Answer from the drawing. Dimensions are ordinates in mm from the lowest x, y and z of the part. A direction names the side the tool comes from. Give positions to 0.01 mm unless a question says otherwise; leave off trailing zeros. Loops run counter-clockwise (first coordinate to the right, second up) from the corner with the lowest first, then second, coordinate; pieces in that order, holes last.
(1) Straight lines are drawn through the part: probe 1 along Z at (x, y) = (92.5, 16.5); probe 2 along Z at (x, y) = (6.5, 30); probe 3 along Y at (x, z) = (22, 6) (1 decimal). For each, find the intervals that lie inside material, in ascending order.
(2) Find section A-A, the plane z = 11. Write down the section's boundary in (x, y), then the cut area to 3 significant figures.
(3) Find section B-B, the plane x = 22.5. Write down the section's boundary in (y, z).
(4) Find section C-C, the plane y = 37.5. Write down the section's boundary in (x, z).
(5) Determine the mould class of the marked faces 1, 2, 3 and 4 for opening direction Y: pulls with the +Y half, pulls with the -Y half, needs draft (parallel to the pull), parting line crosses it, or undercut.
(6) Each of these flat-tipped pins is pushed along its axis until it touches: P1, Ø1, axis at y = 74.5, z = 85, coming from the -X side; P2, Ø15, axis at x = 97.5, y = 8.5, coming from the -Z side. Where does it stop, or does it pass through?
(7) Which of the six approach directions +Z, -Z, +X, -X, +Y, -Y give full straight-line access (tool end or side, diameter ignored) to the marked faces 5, 6 and 7?
(8) Find section D-D, the plane x = 120.5. Write down the section's boundary in (y, z), then the cut area to 3 significant figures.
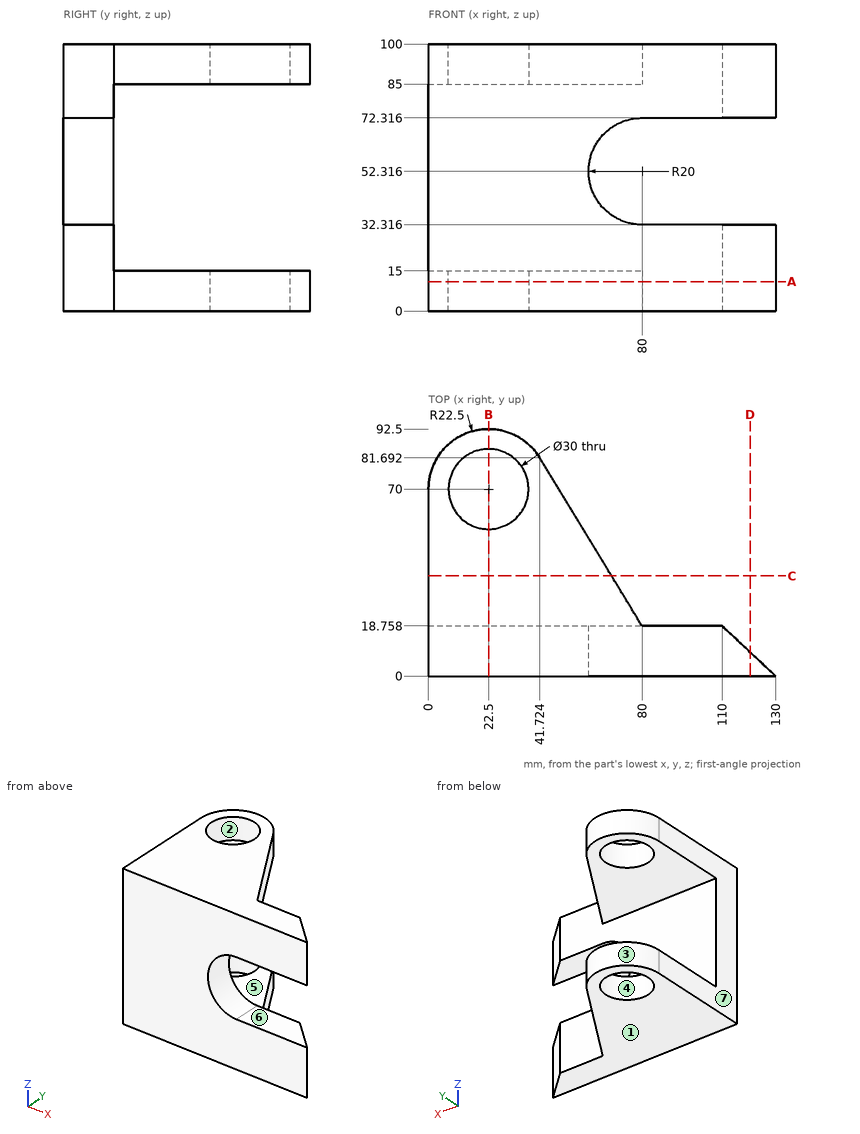
Entries:
1. probe 1: z = 0 to 32.32, 72.32 to 100
1. probe 2: z = 0 to 15, 85 to 100
1. probe 3: y = 0 to 55, 85 to 92.5
2. outline: (0, 0) - (130, 0) - (110, 18.76) - (80, 18.76) - (41.72, 81.69) arc R22.5 ccw to (0, 70) - close; hole circle Ø30 at (22.5, 70)
2. area: 5,660 mm2
3. outline: (0, 0) - (55, 0) - (55, 15) - (18.76, 15) - (18.76, 85) - (55, 85) - (55, 100) - (0, 100) - close; (85, 0) - (92.5, 0) - (92.5, 15) - (85, 15) - close; (85, 85) - (92.5, 85) - (92.5, 100) - (85, 100) - close
4. outline: (0, 0) - (68.6, 0) - (68.6, 15) - (0, 15) - close; (0, 85) - (68.6, 85) - (68.6, 100) - (0, 100) - close
5. face 1: needs draft
5. face 2: undercut
5. face 3: pulls with the +Y half
5. face 4: undercut
6. P1: stops at x = 0.36
6. P2: stops at z = 0
7. face 5: +X, -X, +Y
7. face 6: +X, +Y, -Y
7. face 7: +Z, -Z, -X, +Y, -Y
8. outline: (0, 0) - (8.91, 0) - (8.91, 32.32) - (0, 32.32) - close; (0, 72.32) - (8.91, 72.32) - (8.91, 100) - (0, 100) - close
8. area: 535 mm2
